```python
from build123d import *

# Parameters (mm, degrees)
F0_W      = 46.482
F0_H      = 25.4
F1_DEPTH  = 23.622
F2_W      = 16.59
F2_H      = 25.4
F2_W_2    = 5
F3_DEPTH  = 10
F4_W      = 6
F4_H      = 18
F5_DEPTH  = 13.623
F6_W      = 30
F6_H      = 3
F7_DEPTH  = 25.401
F8_R      = 1.5875
F9_DEPTH  = 10
F10_R     = 3
F11_DEPTH = 1
F12_SIZE  = 1


with BuildPart() as f1:
    # F0 (on Top) → F1 (new body)
    with BuildSketch(Plane.XY):
        Rectangle(F0_W, F0_H)
    extrude(amount=F1_DEPTH)

    # F2 (on face) → F3 (cut)
    with BuildSketch(Plane.XY.offset(23.622)):
        with Locations((-14.946, 0)):
            Rectangle(F2_W, F2_H)
        with Locations((20.741, 0)):
            Rectangle(F2_W_2, F2_H)
    extrude(amount=-F3_DEPTH, mode=Mode.SUBTRACT)

    # F4 (on face) → F5 (cut, through all)
    with BuildSketch(Plane.XY.offset(13.622)):
        with Locations((-20.241, 0)):
            Rectangle(F4_W, F4_H)
    extrude(amount=-F5_DEPTH, mode=Mode.SUBTRACT)

    # F6 (on face) → F7 (cut, through all)
    with BuildSketch(Plane(origin=(0, 12.7, 0), x_dir=(-1, 0, 0), z_dir=(0, 1, 0))):
        with Locations((1.759, 1.5)):
            Rectangle(F6_W, F6_H)
    extrude(amount=-F7_DEPTH, mode=Mode.SUBTRACT)

    # F8 (on face) → F9 (join)
    with BuildSketch(Plane(origin=(-6.651, 0, 0), x_dir=(0, -1, 0), z_dir=(-1, 0, 0))):
        with Locations((-6.35, 18.622)):
            Circle(F8_R)
        with Locations((6.35, 18.622)):
            Circle(F8_R)
    extrude(amount=F9_DEPTH)

    # F10 (on face) → F11 (join)
    with BuildSketch(Plane(origin=(-6.651, 0, 0), x_dir=(0, -1, 0), z_dir=(-1, 0, 0))):
        with Locations((-6.35, 18.622)):
            Circle(F10_R)
        with Locations((6.35, 18.622)):
            Circle(F10_R)
    extrude(amount=F11_DEPTH)

    # F12
    f12_edges = [f1.edges().sort_by_distance(p)[0] for p in [
        (-16.651, 7.9375, 18.622),
        (-16.651, -4.7625, 18.622),
    ]]
    chamfer(f12_edges, length=F12_SIZE)


solid = f1.part
```
The listing builds one solid part. Answer for the finished solid, in the listing's coordinates (mm). A direction names the side the tool comes from. Give positions to 0.01 mm unless a question says otherwise; leave off trailing zeros. Order: outer loops, then holes, each group sorted by start corner. A loop starts at its lowest first (then second) coordinate and runs counter-clockwise, first axis right, second up. Notation, with made-up numbers: M -13.5,17 L -1.5,17 A21 cw -1.5,53 Z; hole C 59.5,-20 d6. An arc over 180 degrees is marked long. Put each result on its own line as item: value. Start each with the question number.
Item 1: Find the intervals of material crossed by line 1 along Z through (x, y) = (19.5, -10); line 2 along X through (y, z) = (2.75, 10.75); line 3 along Z through (x, y) = (-6.5, 5.5), in increasing order.
Item 2: The part is cut by section A-A, the plane x = -20. Determine the outline of the cut face in (y, z), and give its area (3 significant figures).
Item 3: The part is cut by section B-B, the plane y = 6.35. Determine the outline of the cut face in (x, z), and give its area (3 significant figures).
Item 4: The part is cut by section D-D, the plane x = -8.5. State how many separate pieces and enclosed holes the cut face has, and give its area (3 significant figures).
Item 5: For a pull along Z with two mould halves and no side action, classify faces 1 (the face through (21, 0, 13.622)), 2 (the face through (-7.1, 6.7, 21.6)), 3 (the face through (23.241, 0, 7)) as +Z half, -Z half, draft (parallel to the pull), parting line (faces both ways), or undercut.
Item 6: Flat-ended cylindrical pins translate along their axes: P1, Ø3, axis at y = -1.5, z = 17.5, coming from the +X side; P2, Ø3, axis at y = -2, z = 18.5, coming from the -X side; P3, Ø2.5, axis at x = 20, y = -5.5, coming from the +Z side. Find the tip coordinate at first contact, or state that the pin passes through.
Item 7: Which of the six approach directions +Z, -Z, +X, -X, +Y, -Y give full straight-line access (tool end or side, diameter ignored) to faces 4 (the face through (-16.651, 6.4, 18.6)), 5 (the face through (-11.595, -6.143, 20.196)), 6 (the face through (13.241, 0, 1))?
Item 8: The part is cut by section C-C, the plane z = 5.5. Determine the outline of the cut face in (x, y), and give its area (3 significant figures).
Answer key:
1. line 1: z = 0 to 13.62
1. line 2: x = -17.24 to 23.24
1. line 3: z = 3 to 23.62
2. outline: M -12.7,0 L -9,0 L -9,13.62 L -12.7,13.62 Z; M 9,0 L 12.7,0 L 12.7,13.62 L 9,13.62 Z
2. area: 101 mm²
3. outline: M -17.24,0 L -16.76,0 L -16.76,3 L 13.24,3 L 13.24,0 L 23.24,0 L 23.24,13.62 L 18.24,13.62 L 18.24,23.62 L -6.65,23.62 L -6.65,21.62 L -7.65,21.62 L -7.65,20.21 L -15.65,20.21 L -16.65,19.21 L -16.65,18.03 L -15.65,17.03 L -7.65,17.03 L -7.65,15.62 L -6.65,15.62 L -6.65,13.62 L -17.24,13.62 Z
3. area: 744 mm²
4. separate pieces: 3
4. enclosed holes: 0
4. area: 286 mm²
5. face 1: +Z half
5. face 2: undercut
5. face 3: draft
6. P1: stops at x = 18.24
6. P2: stops at x = -7.65
6. P3: stops at z = 13.62
7. face 4: +Z, -X, +Y, -Y
7. face 5: -X
7. face 6: -Z, +Y, -Y
8. outline: M -23.24,-12.7 L 23.24,-12.7 L 23.24,12.7 L -23.24,12.7 L -23.24,9 L -17.24,9 L -17.24,-9 L -23.24,-9 Z
8. area: 1,070 mm²
